Work out the finished part from the listing and answer in its coordinate system (mm). Face numbers are marked on the shaded views. A direction names the side the tool comes from. Round coordinates to 2 decimals unless told otherwise and drop trailing zeros. Order: outer loops, then holes, each group sorted by start corner. A loop starts at its lowest first (then second) coordinate and runs counter-clockwise, first axis right, second up.
Autodesk Inventor part; units mm, degrees
ref_plane "YZ Plane" through (0, 0, 0) normal (1, 0, 0) x (0, 1, 0)
ref_plane "XZ Plane" through (0, 0, 0) normal (0, 1, 0) x (-1, 0, 0)
ref_plane "XY Plane" through (0, 0, 0) normal (0, 0, 1) x (1, 0, 0)
sketch "Sketch1" plane through (0, 0, 0) normal (0, 0, 1) x (1, 0, 0)
  line L0 (-10, 43.5021) -> (10, 43.5021)
  line L1 (10, 43.5021) -> (10, -36.4979)
  line L2 (10, -36.4979) -> (-10, -36.4979)
  line L3 (-10, -36.4979) -> (-10, 43.5021)
  arc A0 (-10, -59.7738) -> (10, -36.4979) centre (-19.0329, -31.7817) ccw
  line L4 (-10, -59.7738) -> (-10, -36.4979)
  point P0 (0, 0)
  dimension "d0" = 20
  dimension "d1" = 10
  dimension "d2" = 80
extrude "Extrusion1" add sketch "Sketch1" along normal blind 10
sketch "Sketch2" plane through (0, 0, 10) normal (0, 0, 1) x (1, 0, 0)
  line L0 (-10, 43.5021) -> (-10, -59.7738)
  line L1 (-10, 33.5021) -> (10, 33.5021)
  line L2 (10, 33.5021) -> (10, 58.8152)
  line L3 (-10, 58.8152) -> (-10, 33.5021)
  line L4 (10, 43.5021) -> (-10, 43.5021)
  arc A0 (10, 58.8152) -> (-10, 58.8152) centre (0, 58.8152) ccw
  circle A1 centre (0, 58.8152) radius 5
  point P0 (0, 0)
  dimension "d5" = 20
  dimension "d6" = 10
  dimension "d7" = 10
extrude "Extrusion2" add sketch "Sketch2" along normal blind 10
sketch "Sketch3" plane through (0, 0, 0) normal (0, 0, -1) x (-1, 0, 0)
  point P0 (0, 0)
sketch "Sketch4" plane through (0, 0, 0) normal (0, 0, -1) x (-1, 0, 0)
  line L0 (-10, -36.4979) -> (-10, 43.5021)
  arc A0 (10, 58.8152) -> (-10, 58.8152) centre (0, 58.8152) ccw
  line L1 (-10, 33.5021) -> (10, 33.5021)
  line L2 (10, 33.5021) -> (10, 58.8152)
  line L3 (-10, 58.8152) -> (-10, 33.5021)
  line L4 (-10, 43.5021) -> (10, 43.5021)
  arc A1 (10, 58.8152) -> (-10, 58.8152) centre (0, 58.8152) ccw
  circle A2 centre (0, 58.8152) radius 5
  point P0 (0, 0)
  point P1 (-10, 58.8152)
  dimension "d10" = 10
extrude "Extrusion3" add sketch "Sketch4" along normal blind 10
properties part number "foot"
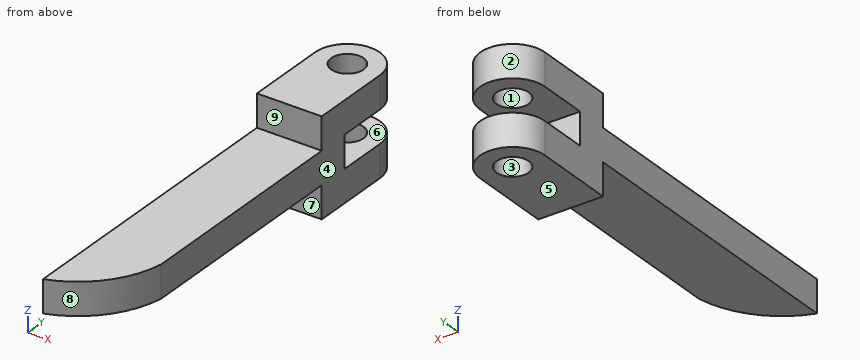
Item 1: For a pull along Y with two mould halves and no side action, classify the marked faces 1, 2, 3 and 4 as released by +Y, released by -Y, zero draft, split by the parting line, or undercut.
Item 2: Given pin 1 (10 mm diameter, centred on x = 5.5, z = 5, fed in from -Y); pin 2 (9 mm diameter, centred on x = 0, y = 58.82, fed in from +Z); pin 3 (8 mm diameter, centred on x = -1, z = -5.5, fed in from -Y); pin 4 (3 mm diameter, centred on x = -4.5, z = 4.5, fed in from +Y), each flat-ended and moving along its own axis, determine where each tip first touches the part or whether it passes through.
Item 3: Find section A-A (z = -3.5). Write down the section's boundary in (x, y).
Item 4: Find section C-C (y = 18). Write down the section's boundary in (x, z), plus the area to 3 significant figures.
Item 5: Find the intervals of material crossed by line 1 along Z through (x, y) = (-5.25, 60.5); line 2 along Y through (x, z) = (0, 12.5); line 3 along Z through (x, y) = (-8.5, 16.5), in increasing order.
Item 6: A tool of negligible diameter and unlimited length cuts with its end or side. For the marked faces 5, 6, 7, 8 and 9, from which of +Z, -Z, +X, -X, +Y, -Y can it reach the whole face along a straight path? Write none if from no direction.
Item 7: Find section D-D (z = 6.25). Write down the section's boundary in (x, y).
Item 8: Find section B-B (x = -2.75). Write down the section's boundary in (y, z), plus the area to 3 significant figures.
Model answer:
1. face 1: undercut
1. face 2: released by +Y
1. face 3: undercut
1. face 4: zero draft
2. pin 1: stops at y = -53.77
2. pin 2: passes through
2. pin 3: stops at y = 33.5
2. pin 4: stops at y = 43.5
3. outline: (-10, 33.5) - (10, 33.5) - (10, 58.82) arc R10 ccw to (-10, 58.82) - close; hole circle Ø10 at (0, 58.82)
4. outline: (-10, 0) - (10, 0) - (10, 10) - (-10, 10) - close
4. area: 200 mm2
5. line 1: z = -10 to 0, 10 to 20
5. line 2: y = 33.5 to 53.82, 63.82 to 68.82
5. line 3: z = 0 to 10
6. face 5: -Z, +X, -X, +Y, -Y
6. face 6: +X, -X, +Y
6. face 7: -Z, +X, -X, -Y
6. face 8: +Z, -Z, +X, -Y
6. face 9: +Z, +X, -X, -Y
7. outline: (-10, -59.77) arc R29.41 ccw to (10, -36.5) - (10, 43.5) - (-10, 43.5) - close
8. outline: (-56.28, 0) - (33.5, 0) - (33.5, -10) - (54.64, -10) - (54.64, 0) - (43.5, 0) - (43.5, 10) - (54.64, 10) - (54.64, 20) - (33.5, 20) - (33.5, 10) - (-56.28, 10) - close; (62.99, -10) - (68.43, -10) - (68.43, 0) - (62.99, 0) - close; (62.99, 10) - (68.43, 10) - (68.43, 20) - (62.99, 20) - close
8. area: 1,530 mm2
